```python
from build123d import *

# Parameters (mm, degrees)
BOSS_EXTRUDE1_DEPTH = 5
SKETCH2_R           = 5
CUT_EXTRUDE1_DEPTH  = 178.411949992
SKETCH5_R           = 2.5
CUT_EXTRUDE4_DEPTH  = 12.5
CUT_EXTRUDE5_DEPTH  = 10
SKETCH7_R           = 2.5
CUT_EXTRUDE6_DEPTH  = 10
SKETCH8_R           = 2.5
CUT_EXTRUDE7_DEPTH  = 10
SKETCH9_R           = 8.75
CUT_EXTRUDE8_DEPTH  = 2.5
SKETCH10_W          = 230
SKETCH10_H          = 135
CUT_EXTRUDE9_DEPTH  = 10


with BuildPart() as part:
    # Sketch1 → Boss-Extrude1 (new body)
    with BuildSketch(Plane.XY):
        with BuildLine():
            ThreePointArc((108.79085436, -12.15404787), (115, 0), (108.79085436, 12.15404787))
            ThreePointArc((108.79085436, 12.15404787), (68.702723984, 59.351361992), (54.997750912, 119.740254766))
            ThreePointArc((54.997750912, 119.740254766), (48.179588548, 132.573556823), (33.684210526, 133.60554311))
            ThreePointArc((33.684210526, 133.60554311), (0, 126.168439698), (-33.684210526, 133.60554311))
            ThreePointArc((-33.684210526, 133.60554311), (-48.179588548, 132.573556823), (-54.997750912, 119.740254766))
            ThreePointArc((-54.997750912, 119.740254766), (-68.702723984, 59.351361992), (-108.79085436, 12.15404787))
            ThreePointArc((-108.79085436, 12.15404787), (-115, 0), (-108.79085436, -12.15404787))
            ThreePointArc((-108.79085436, -12.15404787), (-68.702723984, -59.351361992), (-54.997750912, -119.740254766))
            ThreePointArc((-54.997750912, -119.740254766), (-48.179588548, -132.573556823), (-33.684210526, -133.60554311))
            ThreePointArc((-33.684210526, -133.60554311), (0, -126.168439698), (33.684210526, -133.60554311))
            ThreePointArc((33.684210526, -133.60554311), (48.179588548, -132.573556823), (54.997750912, -119.740254766))
            ThreePointArc((54.997750912, -119.740254766), (68.702723984, -59.351361992), (108.79085436, -12.15404787))
        make_face()
    extrude(amount=BOSS_EXTRUDE1_DEPTH)

    # Sketch2 → Cut-Extrude1 (cut, through all)
    with BuildSketch(Plane(origin=(0, 0, 0), x_dir=(-1, 0, 0), z_dir=(0, 0, -1))):
        with Locations((-40, 120)):
            Circle(SKETCH2_R)
        with Locations((-100, 0)):
            Circle(SKETCH2_R)
        with Locations(Location((100, 0, 0), (0, 0, 180))):
            Circle(SKETCH2_R)
        with Locations(Location((40, 120, 0), (0, 0, 180))):
            Circle(SKETCH2_R)
        with Locations((40, -120)):
            Circle(SKETCH2_R)
        with Locations(Location((-40, -120, 0), (0, 0, 180))):
            Circle(SKETCH2_R)
    extrude(amount=-CUT_EXTRUDE1_DEPTH, mode=Mode.SUBTRACT)

    # Sketch5 → Cut-Extrude4 (cut)
    with BuildSketch(Plane(origin=(0, 0, 0), x_dir=(-1, 0, 0), z_dir=(0, 0, -1))):
        with Locations((20, 95)):
            Circle(SKETCH5_R)
        with Locations((0, 95)):
            Circle(SKETCH5_R)
        with Locations((10, 95)):
            Circle(SKETCH5_R)
        with Locations(Location((10, -95, 0), (0, 0, 180))):
            Circle(SKETCH5_R)
        with Locations(Location((0, -95, 0), (0, 0, 180))):
            Circle(SKETCH5_R)
        with Locations(Location((20, -95, 0), (0, 0, 180))):
            Circle(SKETCH5_R)
        with Locations(Location((-20, 95, 0), (0, 0, 180))):
            Circle(SKETCH5_R)
        with Locations(Location((-10, 95, 0), (0, 0, 180))):
            Circle(SKETCH5_R)
        with Locations((-20, -95)):
            Circle(SKETCH5_R)
        with Locations((-10, -95)):
            Circle(SKETCH5_R)
    extrude(amount=-CUT_EXTRUDE4_DEPTH, mode=Mode.SUBTRACT)

    # Sketch6 → Cut-Extrude5 (cut)
    with BuildSketch(Plane.XY.offset(5)):
        with BuildLine():
            Line((42.5, 75), (42.5, 45))
            ThreePointArc((42.5, 45), (40, 42.5), (37.5, 45))
            Line((37.5, 45), (37.5, 75))
            ThreePointArc((37.5, 75), (40, 77.5), (42.5, 75))
        make_face()
        with BuildLine():
            Line((22.5, 75), (22.5, 45))
            ThreePointArc((22.5, 45), (20, 42.5), (17.5, 45))
            Line((17.5, 45), (17.5, 75))
            ThreePointArc((17.5, 75), (20, 77.5), (22.5, 75))
        make_face()
        with BuildLine():
            Line((2.5, 75), (2.5, 45))
            ThreePointArc((2.5, 45), (0, 42.5), (-2.5, 45))
            Line((-2.5, 45), (-2.5, 75))
            ThreePointArc((-2.5, 75), (0, 77.5), (2.5, 75))
        make_face()
        with BuildLine():
            Line((-17.5, 75), (-17.5, 45))
            ThreePointArc((-17.5, 45), (-20, 42.5), (-22.5, 45))
            Line((-22.5, 45), (-22.5, 75))
            ThreePointArc((-22.5, 75), (-20, 77.5), (-17.5, 75))
        make_face()
        with BuildLine():
            Line((-37.5, 75), (-37.5, 45))
            ThreePointArc((-37.5, 45), (-40, 42.5), (-42.5, 45))
            Line((-42.5, 45), (-42.5, 75))
            ThreePointArc((-42.5, 75), (-40, 77.5), (-37.5, 75))
        make_face()
        with BuildLine():
            Line((42.5, 15), (42.5, -15))
            ThreePointArc((42.5, -15), (40, -17.5), (37.5, -15))
            Line((37.5, -15), (37.5, 15))
            ThreePointArc((37.5, 15), (40, 17.5), (42.5, 15))
        make_face()
        with BuildLine():
            Line((22.5, 15), (22.5, -15))
            ThreePointArc((22.5, -15), (20, -17.5), (17.5, -15))
            Line((17.5, -15), (17.5, 15))
            ThreePointArc((17.5, 15), (20, 17.5), (22.5, 15))
        make_face()
        with BuildLine():
            Line((2.5, 15), (2.5, -15))
            ThreePointArc((2.5, -15), (0, -17.5), (-2.5, -15))
            Line((-2.5, -15), (-2.5, 15))
            ThreePointArc((-2.5, 15), (0, 17.5), (2.5, 15))
        make_face()
        with BuildLine():
            Line((-17.5, 15), (-17.5, -15))
            ThreePointArc((-17.5, -15), (-20, -17.5), (-22.5, -15))
            Line((-22.5, -15), (-22.5, 15))
            ThreePointArc((-22.5, 15), (-20, 17.5), (-17.5, 15))
        make_face()
        with BuildLine():
            Line((-37.5, 15), (-37.5, -15))
            ThreePointArc((-37.5, -15), (-40, -17.5), (-42.5, -15))
            Line((-42.5, -15), (-42.5, 15))
            ThreePointArc((-42.5, 15), (-40, 17.5), (-37.5, 15))
        make_face()
        with BuildLine():
            Line((42.5, -45), (42.5, -75))
            ThreePointArc((42.5, -75), (40, -77.5), (37.5, -75))
            Line((37.5, -75), (37.5, -45))
            ThreePointArc((37.5, -45), (40, -42.5), (42.5, -45))
        make_face()
        with BuildLine():
            Line((22.5, -45), (22.5, -75))
            ThreePointArc((22.5, -75), (20, -77.5), (17.5, -75))
            Line((17.5, -75), (17.5, -45))
            ThreePointArc((17.5, -45), (20, -42.5), (22.5, -45))
        make_face()
        with BuildLine():
            Line((2.5, -45), (2.5, -75))
            ThreePointArc((2.5, -75), (0, -77.5), (-2.5, -75))
            Line((-2.5, -75), (-2.5, -45))
            ThreePointArc((-2.5, -45), (0, -42.5), (2.5, -45))
        make_face()
        with BuildLine():
            Line((-17.5, -45), (-17.5, -75))
            ThreePointArc((-17.5, -75), (-20, -77.5), (-22.5, -75))
            Line((-22.5, -75), (-22.5, -45))
            ThreePointArc((-22.5, -45), (-20, -42.5), (-17.5, -45))
        make_face()
        with BuildLine():
            Line((-37.5, -45), (-37.5, -75))
            ThreePointArc((-37.5, -75), (-40, -77.5), (-42.5, -75))
            Line((-42.5, -75), (-42.5, -45))
            ThreePointArc((-42.5, -45), (-40, -42.5), (-37.5, -45))
        make_face()
    extrude(amount=-CUT_EXTRUDE5_DEPTH, mode=Mode.SUBTRACT)

    # Sketch7 → Cut-Extrude6 (cut)
    with BuildSketch(Plane.XY.offset(5)):
        with Locations((-65, 30)):
            Circle(SKETCH7_R)
        with Locations((-55, 30)):
            Circle(SKETCH7_R)
        with Locations((-45, 30)):
            Circle(SKETCH7_R)
        with Locations((-35, 30)):
            Circle(SKETCH7_R)
        with Locations((-25, 30)):
            Circle(SKETCH7_R)
        with Locations((-15, 30)):
            Circle(SKETCH7_R)
        with Locations((-5, 30)):
            Circle(SKETCH7_R)
        with Locations((5, 30)):
            Circle(SKETCH7_R)
        with Locations((15, 30)):
            Circle(SKETCH7_R)
        with Locations((25, 30)):
            Circle(SKETCH7_R)
        with Locations((35, 30)):
            Circle(SKETCH7_R)
        with Locations((45, 30)):
            Circle(SKETCH7_R)
        with Locations((55, 30)):
            Circle(SKETCH7_R)
        with Locations((65, 30)):
            Circle(SKETCH7_R)
        with Locations((65, -30)):
            Circle(SKETCH7_R)
        with Locations((55, -30)):
            Circle(SKETCH7_R)
        with Locations((45, -30)):
            Circle(SKETCH7_R)
        with Locations((35, -30)):
            Circle(SKETCH7_R)
        with Locations((25, -30)):
            Circle(SKETCH7_R)
        with Locations((15, -30)):
            Circle(SKETCH7_R)
        with Locations((5, -30)):
            Circle(SKETCH7_R)
        with Locations((-5, -30)):
            Circle(SKETCH7_R)
        with Locations((-15, -30)):
            Circle(SKETCH7_R)
        with Locations((-25, -30)):
            Circle(SKETCH7_R)
        with Locations((-35, -30)):
            Circle(SKETCH7_R)
        with Locations((-45, -30)):
            Circle(SKETCH7_R)
        with Locations((-55, -30)):
            Circle(SKETCH7_R)
        with Locations((-65, -30)):
            Circle(SKETCH7_R)
    extrude(amount=-CUT_EXTRUDE6_DEPTH, mode=Mode.SUBTRACT)

    # Sketch8 → Cut-Extrude7 (cut)
    with BuildSketch(Plane.XY.offset(5)):
        with Locations((-65, 0)):
            Circle(SKETCH8_R)
        with Locations((-65, 15)):
            Circle(SKETCH8_R)
        with Locations((-65, -15)):
            Circle(SKETCH8_R)
        with Locations((65, -15)):
            Circle(SKETCH8_R)
        with Locations((65, 0)):
            Circle(SKETCH8_R)
        with Locations((65, 15)):
            Circle(SKETCH8_R)
    extrude(amount=-CUT_EXTRUDE7_DEPTH, mode=Mode.SUBTRACT)

    # Sketch9 → Cut-Extrude8 (cut)
    with BuildSketch(Plane(origin=(0, 0, 0), x_dir=(-1, 0, 0), z_dir=(0, 0, -1))):
        with Locations((100, 0)):
            Circle(SKETCH9_R)
        with Locations((40, 120)):
            Circle(SKETCH9_R)
        with Locations((40, -120)):
            Circle(SKETCH9_R)
        with Locations((-40, -120)):
            Circle(SKETCH9_R)
        with Locations((-100, 0)):
            Circle(SKETCH9_R)
        with Locations((-40, 120)):
            Circle(SKETCH9_R)
    extrude(amount=-CUT_EXTRUDE8_DEPTH, mode=Mode.SUBTRACT)

    # Sketch10 → Cut-Extrude9 (cut)
    with BuildSketch(Plane.XY.offset(5)):
        with Locations((0, 67.5)):
            Rectangle(SKETCH10_W, SKETCH10_H)
    extrude(amount=-CUT_EXTRUDE9_DEPTH, mode=Mode.SUBTRACT)


solid = part.part
```
The model under review builds one solid part; all positions refer to its coordinate system, in mm. A direction names the side the tool comes from. Round coordinates to 2 decimals unless told otherwise and drop trailing zeros. Order: outer loops, then holes, each group sorted by start corner. A loop starts at its lowest first (then second) coordinate and runs counter-clockwise, first axis right, second up. Notation, with made-up numbers: (73.5, 35.25) -> (100.5, 35.25) arc R22 ccw to (100.5, 58.25) -> close; hole circle Ø3 at (2.25, 34). An arc over 180 degrees is marked (long way). Use a Markdown table: item, result.
Q1. Clearance check with flat-ended pins moving along their axes: P1, Ø2.5, axis at y = -66, z = 1.5, coming from the -X side; P2, Ø2, axis at y = -75, z = 1, coming from the -X side; P3, Ø4, axis at x = -25, y = -30, coming from the -Z side; P4, Ø2, axis at y = -100.5, z = 2, coming from the +X side. State where each tip first meets the part, or that it passes through.
Values:
| item | result |
|---|---|
| P1 | stops at x = -66.16 |
| P2 | stops at x = -62.47 |
| P3 | passes through |
| P4 | stops at x = 56.23 |
Q2. We need section C-C on x = -15. Write out the cut boundary in (y, z), then the cut area to 3 significant figures.
Values:
| item | result |
|---|---|
| outline | (-127.59, 0) -> (-32.5, 0) -> (-32.5, 5) -> (-127.59, 5) -> close; (-27.5, 0) -> (0, 0) -> (0, 5) -> (-27.5, 5) -> close |
| area | 613 mm^2 |
Q3. We need section B-B on y = -61. Write out the cut boundary in (x, z), then the cut area to 3 significant figures.
Values:
| item | result |
|---|---|
| outline | (-67.89, 0) -> (-42.5, 0) -> (-42.5, 5) -> (-67.89, 5) -> close; (-37.5, 0) -> (-22.5, 0) -> (-22.5, 5) -> (-37.5, 5) -> close; (-17.5, 0) -> (-2.5, 0) -> (-2.5, 5) -> (-17.5, 5) -> close; (2.5, 0) -> (17.5, 0) -> (17.5, 5) -> (2.5, 5) -> close; (22.5, 0) -> (37.5, 0) -> (37.5, 5) -> (22.5, 5) -> close; (42.5, 0) -> (67.89, 0) -> (67.89, 5) -> (42.5, 5) -> close |
| area | 554 mm^2 |
Q4. Tool access review of faces 4 (the flat face through (100.1, -5.3, 2.5)), 5 (the flat face through (-53, 0, 3)), 6 (the cylindrical face through (-19.9, -77.5, 2.5)), 7 (the flat face through (-37.5, -7, 3)): name each direction out of +Z, -Z, +X, -X, +Y, -Y from which nothing blocks a thin tool from reaching the whole face with its end or side.
Values:
| item | result |
|---|---|
| face 4 | -Z, +Y |
| face 5 | +Z, -Z, +X, -X, +Y |
| face 6 | +Z, -Z |
| face 7 | +Z, -Z, +Y |
Q5. Mouldability with a two-part tool opening along Y and no side actions: class faces 1 (the flat face through (2.5, -60, 3)), 2 (the flat face through (-30, 0, 3)), 3 (the flat face through (22.5, -7, 3)) as +Y half, -Y half, draft (parallel to the pull), parting line (faces both ways), or undercut.
Values:
| item | result |
|---|---|
| face 1 | undercut |
| face 2 | +Y half |
| face 3 | draft |
Q6. We need section D-D on x = 100. Write out the cut boundary in (y, z).
Values:
| item | result |
|---|---|
| outline | (-19.11, 0) -> (-8.75, 0) -> (-8.75, 2.5) -> (-5, 2.5) -> (-5, 5) -> (-19.11, 5) -> close |
Q7. We need section A-A on x = 20. Write out the cut boundary in (y, z).
Values:
| item | result |
|---|---|
| outline | (-128.71, 0) -> (-97.5, 0) -> (-97.5, 5) -> (-128.71, 5) -> close; (-92.5, 0) -> (-77.5, 0) -> (-77.5, 5) -> (-92.5, 5) -> close; (-42.5, 0) -> (-17.5, 0) -> (-17.5, 5) -> (-42.5, 5) -> close |
Q8. For line 1 (X direction, y = -73.5, z = 1.15); line 2 (Y direction, x = 44.5, z = 4.5); line 3 (X direction, y = -116, z = 2.2), list the stretches that pass through material, from the lowest coordinate up.
Values:
| item | result |
|---|---|
| line 1 | x = -62.65 to -42.5, -37.5 to -22.5, -17.5 to -2.5, 2.5 to 17.5, 22.5 to 37.5, 42.5 to 62.65 |
| line 2 | y = -134.31 to -122.18, -117.82 to -32.45, -27.55 to 0 |
| line 3 | x = -54.99 to -47.78, -32.22 to 32.22, 47.78 to 54.99 |
